The drawing under review shows one solid part. Ordinate dimensions are in mm from its lowest x, y, z. Round coordinates to 2 decimals unless told otherwise and drop trailing zeros. Write each loop counter-clockwise with the first axis right and the second up, starting at its lowest first coordinate (ties: lowest second). Pieces come first, ordered by that corner, then holes. Notation, with made-up numbers: M -8,-1.5 L 25,-1.5 A10 cw 25,4.5 Z; hole C 28,17.5 d6. An arc over 180 degrees is marked long. Write item = value, one per line. Start each with the question number.
Item 1: Take a section at A-A, the plane x = 31.5. Give the boundary of the cut face in (y, z).
Item 2: Take a section at C-C, the plane y = 2.5. Give the boundary of the cut face in (x, z), plus the area to 3 significant figures.
Item 3: Take a section at B-B, the plane z = 1.75. Give the boundary of the cut face in (x, y).
Item 4: The part is to be moulded in two halves that separate along X. For the marked faces 1, 2 and 3, say which applies: +X half, -X half, draft (parallel to the pull), parting line (faces both ways), or undercut.
Item 5: Take a section at D-D, the plane y = 30.5. Give the boundary of the cut face in (x, z), plus the area to 3 significant figures.
Item 6: To check wall thickness, follow line 1 along Y through (x, z) = (25, 1.5); line 2 along Z through (x, y) = (27, 3); line 3 along Z through (x, y) = (18, 29.5). State the ranges of each line that lie inside material, in increasing order.
Item 7: For pin 1 Ø6 at (y, z) = (28.5, 15) entering from -X, flat-tipped, find the tip position at first contact; note if it passes through.
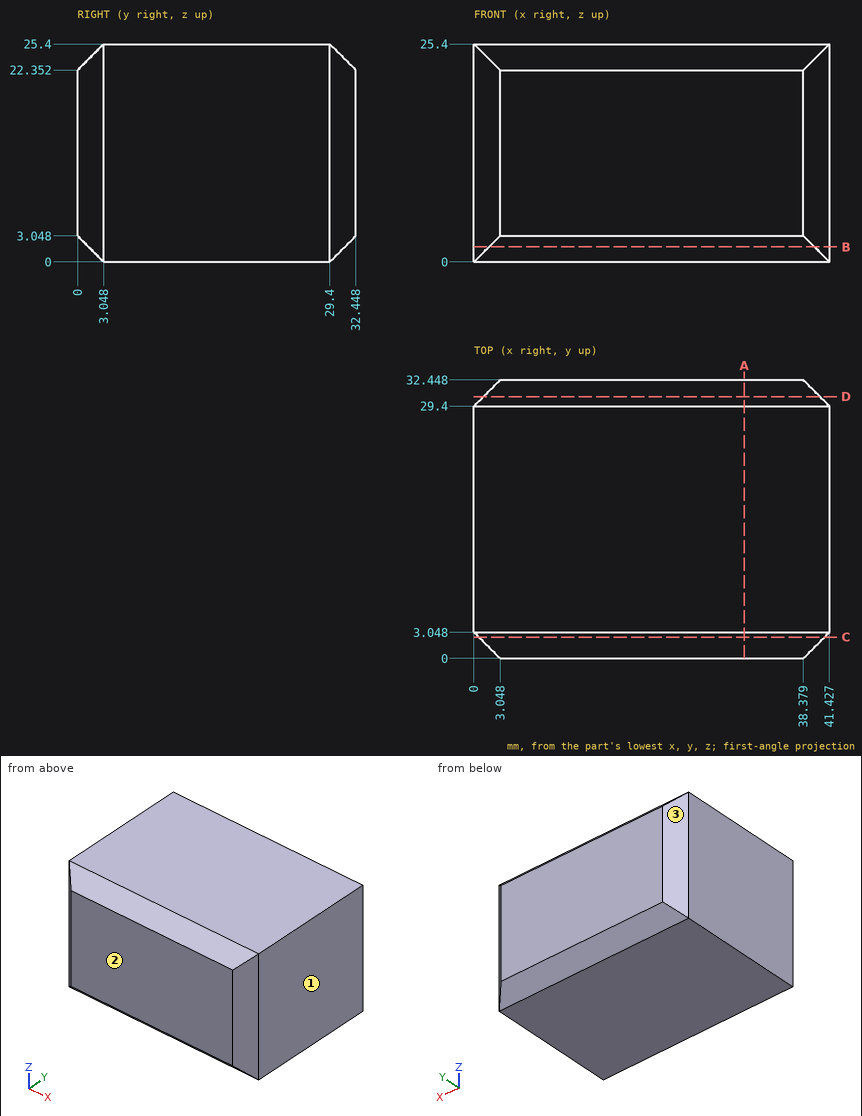
Response values:
q1.outline = M 0,3.05 L 3.05,0 L 29.4,0 L 32.45,3.05 L 32.45,22.35 L 29.4,25.4 L 3.05,25.4 L 0,22.35 Z
q2.outline = M 0.55,0.55 L 40.88,0.55 L 40.88,24.85 L 0.55,24.85 Z
q2.area = 980 mm2
q3.outline = M 0,3.05 L 1.75,1.3 L 39.68,1.3 L 41.43,3.05 L 41.43,29.4 L 39.68,31.15 L 1.75,31.15 L 0,29.4 Z
q4.face_1 = +X half
q4.face_2 = draft
q4.face_3 = -X half
q5.outline = M 1.1,1.1 L 40.33,1.1 L 40.33,24.3 L 1.1,24.3 Z
q5.area = 910 mm2
q6.line_1 = 1.55 to 30.9
q6.line_2 = 0.05 to 25.35
q6.line_3 = 0.1 to 25.3
q7.pin_1 = 0
